Source: CAD feature listing. Evaluate the final solid. Frame: model axes, mm. A direction names the side the tool comes from. Give positions to 0.01 mm unless a question says otherwise; leave off trailing zeros. Loops run counter-clockwise (first coordinate to the right, second up) from the corner with the lowest first, then second, coordinate; pieces in that order, holes last. Notation, with made-up numbers: (67, 66.5) - (105, 66.5) arc R22 cw to (105, 102.5) - close; hole circle Ø7 at (-15.5, 31.5). An arc over 180 degrees is marked (long way). Put each result on its own line as item: value.
```python
from build123d import *

# Parameters (mm, degrees)
SKETCH016_R       = 1.85
EXTRUDE013_DEPTH  = 12
CYLINDER007_R     = 5
CYLINDER007_DEPTH = 1
EXTRUDE012_DEPTH  = 15


with BuildPart() as extrude013:
    # Sketch016 → Extrude013 (new body)
    with BuildSketch(Plane.XZ):
        Polygon((11.75, 36), (11.75, 19), (-13.25, 19), (-19.25, 25), (-19.25, 30), (-13.25, 36), align=None)
        with Locations((-14, 27.481564)):
            Circle(SKETCH016_R, mode=Mode.SUBTRACT)
    extrude(amount=-EXTRUDE013_DEPTH)


with BuildPart() as unprintable:
    # Cylinder007 → Cylinder007 (new body)
    with BuildSketch(Plane(origin=(-14, 18, 27.5), x_dir=(1, 0, 0), z_dir=(0, -1, 0))):
        Circle(CYLINDER007_R)
    extrude(amount=CYLINDER007_DEPTH)


with BuildPart() as body007:
    # Sketch015 → Extrude012 (new body)
    with BuildSketch(Plane.XY.offset(50)):
        with BuildLine():
            ThreePointArc((7.5, 0), (1.009178, 7.431794), (-7.228416, 2))
            Line((-7.228416, 2), (-21.228416, 2))
            Line((-21.228416, 4.25), (-21.228416, 2))
            Line((-8.774964, 4.25), (-21.228416, 4.25))
            ThreePointArc((9.75, 0), (2.180206, 9.503115), (-8.774964, 4.25))
            Line((7.5, 0), (9.75, 0))
        make_face()
    extrude(amount=EXTRUDE012_DEPTH)


with BuildPart() as body007_1:
    # Extrude012 placement: moved
    add(body007.part.moved(Location((0, 0, -30))))

    # Fusion016: union unprintable
    add(unprintable.part)

    # Common001: intersect Extrude013
    add(extrude013.part, mode=Mode.INTERSECT)


with BuildPart() as body007_2:
    # Common001 placement: moved
    add(body007_1.part.moved(Location((1.5, 0, 0))))


with BuildPart() as body007_3:
    # Clone007 placement: moved
    add(body007_2.part.moved(Location((-1.5, 0, 0))))


with BuildPart() as part_mirroring008:
    # Part__Mirroring008: instance of Body007
    add(body007_3.part.mirror(Plane(origin=(0, 0, 0), x_dir=(1, 0, 0), z_dir=(0, 1, 0))))


with BuildPart() as part_mirroring008_1:
    # Part__Mirroring008 placement: moved
    add(part_mirroring008.part.moved(Location((1.5, 0, 0))))


solid = part_mirroring008_1.part
```
1) Section query C-C, the plane z = 34. Output: boundary loops of the cut face in (x, y).
Check result:
outline: (-13.75, -4.25) - (-7.27, -4.25) arc R9.75 ccw to (11.25, 0) - (9, 0) arc R7.5 cw to (-5.73, -2) - (-13.75, -2) - close
2) Access query for faces 1 (the flat face through (-17.75, -3, 27)), 2 (the flat face through (-10, -4.25, 27)), 3 (the flat face through (-10, -2, 27)). Directions: +Z, -Z, +X, -X, +Y, -Y. A direction counts if a zero-diameter tool reaches every point of the face in a straight line with its end or side. Return the directions, or none.
Check result:
face 1: +Z, -Z, -X, +Y, -Y
face 2: +Z, -Z, -X, -Y
face 3: +Z, -Z, -X, +Y
3) Material intervals for line 1 along Z through (x, y) = (-12.5, -3.8); line 2 along X through (y, z) = (-2.5, 27.25); line 3 along Y through (x, z) = (-15.25, 23.5), sorted ascending. Write a range as [from, to].
Check result:
line 1: [20, 25.63], [29.33, 35]
line 2: [-17.75, -14.34], [-10.66, -5.57], [8.57, 10.92]
line 3: [-4.25, -2]
4) Section query B-B, the plane z = 28. Output: boundary loops of the cut face in (x, y).
Check result:
outline: (-17.75, -4.25) - (-14.28, -4.25) - (-14.28, -2) - (-17.75, -2) - close; (-10.72, -4.25) - (-7.27, -4.25) arc R9.75 ccw to (11.25, 0) - (9, 0) arc R7.5 cw to (-5.73, -2) - (-10.72, -2) - close
5) Section query D-D, the plane x = 7.5. Output: boundary loops of the cut face in (y, z).
Check result:
outline: (-7.69, 20) - (-4.5, 20) - (-4.5, 35) - (-7.69, 35) - close
6) Section query A-A, the plane y = -2.75. Output: boundary loops of the cut face in (x, z), plus the area to 3 significant figures.
Check result:
outline: (-17.75, 25) - (-12.75, 20) - (-5.48, 20) - (-5.48, 35) - (-12.75, 35) - (-17.75, 30) - close; (8.48, 20) - (10.85, 20) - (10.85, 35) - (8.48, 35) - close; hole circle Ø3.7 at (-12.5, 27.48)
area: 184 mm²
7) Pin query (flat end, axial travel): P1, Ø1.5, axis at x = -14.5, z = 26, coming from the -Y side; P2, Ø6, axis at x = -12, z = 29.5, coming from the +Y side; P3, Ø5, axis at x = 5, z = 23, coming from the +Y side. Return the tip coordinate at first contact, or that it passes through.
Check result:
P1: y = -4.25
P2: y = -2
P3: y = -4.5
8) Mould query, pull axis Z, two halves, no side actions, for faces 4 (the flat face through (-15.28, -3.11, 32.47)), 5 (the cylindrical face through (-12.901, -3.109, 25.676)), 6 (the cylindrical face through (2.66, -7.41, 27.39)). Classes: pulls with the +Z half, pulls with the -Z half, needs draft (parallel to the pull), parting line crosses it, or undercut.
Check result:
face 4: pulls with the +Z half
face 5: undercut
face 6: needs draft
